```python
from build123d import *

# Parameters (mm, degrees)
EXTRUDE_1_DEPTH     = 3
SKETCH_2_R          = 1.5
CUT_EXTRUDE_1_DEPTH = 3


with BuildPart() as part:
    # 草图1 → 凸台-拉伸1 (new body)
    with BuildSketch(Plane.XY):
        Polygon((0, 0), (15, 0), (32.5, -23), (32.5, -38), (-17.5, -38), (-17.5, -23), align=None)
    extrude(amount=EXTRUDE_1_DEPTH)

    # 草图2 → 切除-拉伸1 (cut)
    with BuildSketch(Plane.XY.offset(3)):
        with Locations((7.5, -4)):
            Circle(SKETCH_2_R)
        with Locations((7.5, -17)):
            Circle(SKETCH_2_R)
        with Locations((28.5, -30.5)):
            Circle(SKETCH_2_R)
        with Locations((-13.5, -30.5)):
            Circle(SKETCH_2_R)
    extrude(amount=-CUT_EXTRUDE_1_DEPTH, mode=Mode.SUBTRACT)


solid = part.part
```
Geometry check sheet. Reference: the model listing, model coordinates, mm. Round coordinates to 2 decimals unless told otherwise and drop trailing zeros. Loops run counter-clockwise (first coordinate to the right, second up) from the corner with the lowest first, then second, coordinate; pieces in that order, holes last. Notation, with made-up numbers: M 31,2 L 79,2 A22 ccw 79,22 Z; hole C -23.5,78 d3. An arc over 180 degrees is marked long. Return JSON: item names as keys, results as strings. Group by question number.
(1) Mould release check, pull along X, two halves, no side actions. Record for faces 1 (the face through (-8.9, -11.7, 1.5)), 2 (the face through (-14.61, -29.49, 1.52)), 3 (the face through (7, 0, 1)): pulls with the +X half, pulls with the -X half, needs draft (parallel to the pull), parting line crosses it, or undercut.
(2) Section check D-D, the plane x = 7.5. Enter the section's corners in (y, z).
(3) Section check A-A, the plane z = 1.15. Enter the section's corners in (x, y), and give its area (3 significant figures).
(4) Section check C-C, the plane y = -4. Enter the section's corners in (x, z).
(5) Go/stop test with flat-tipped pins: pin 1 (5 mm diameter, centred on x = 7.5, y = -17, fed in from +Z); pin 2 (2.5 mm diameter, centred on x = -13.5, y = -30.5, fed in from -Z); pin 3 (1 mm diameter, centred on x = 22.5, z = 1, fed in from +Y). Record where each tip stops, or that it passes through.
(6) Scan lines: line 1 along Y through (x, z) = (7.5, 0.9); line 2 along Y through (x, z) = (7, 1.65); line 3 along X through (y, z) = (-5, 2.3). Record each from-to range of solid material in increasing order. Write a range as [from, to].
(7) Section check B-B, the plane x = -13.5. Enter the section's corners in (y, z).
Data:
{
 "1": {"face 1": "pulls with the -X half", "face 2": "undercut", "face 3": "needs draft"},
 "2": {"outline": "M -38,0 L -18.5,0 L -18.5,3 L -38,3 Z; M -15.5,0 L -5.5,0 L -5.5,3 L -15.5,3 Z; M -2.5,0 L 0,0 L 0,3 L -2.5,3 Z"},
 "3": {"outline": "M -17.5,-38 L 32.5,-38 L 32.5,-23 L 15,0 L 0,0 L -17.5,-23 Z; hole C -13.5,-30.5 d3; hole C 7.5,-17 d3; hole C 7.5,-4 d3; hole C 28.5,-30.5 d3", "area": "1,470 mm²"},
 "4": {"outline": "M -3.04,0 L 6,0 L 6,3 L -3.04,3 Z; M 9,0 L 18.04,0 L 18.04,3 L 9,3 Z"},
 "5": {"pin 1": "z = 3", "pin 2": "through", "pin 3": "y = -9.2"},
 "6": {"line 1": "[-38, -18.5], [-15.5, -5.5], [-2.5, 0]", "line 2": "[-38, -18.41], [-15.59, -5.41], [-2.59, 0]", "line 3": "[-3.8, 6.38], [8.62, 18.8]"},
 "7": {"outline": "M -38,0 L -32,0 L -32,3 L -38,3 Z; M -29,0 L -17.74,0 L -17.74,3 L -29,3 Z"}
}
